Geometry: final body of the model. Coordinates: model frame, mm. A direction names the side the tool comes from. Give positions to 0.01 mm unless a question says otherwise; leave off trailing zeros. Order: outer loops, then holes, each group sorted by start corner. A loop starts at its lowest first (then second) coordinate and runs counter-clockwise, first axis right, second up. Notation, with made-up numbers: (34, -12) -> (48, -12) arc R9 cw to (48, 0) -> close; hole circle Ø11 at (-36, 50). An arc over 180 degrees is marked (long way). One line per question, with ' | ' between items.
Autodesk Inventor part; units mm, degrees
ref_plane "YZ Plane" through (0, 0, 0) normal (1, 0, 0) x (0, 1, 0)
ref_plane "XZ Plane" through (0, 0, 0) normal (0, 1, 0) x (-1, 0, 0)
ref_plane "XY Plane" through (0, 0, 0) normal (0, 0, 1) x (1, 0, 0)
sketch "Skizze1" plane through (0, 0, 0) normal (0, 0, 1) x (1, 0, 0)
  line L0 (0, 0) -> (0, 1.7)
  line L1 (0, 1.7) -> (-5, 1.7)
  line L2 (-5, 1.7) -> (-5, 0.2)
  line L3 (-5, 0.2) -> (-7.5, 0.2)
  line L4 (-7.5, 0.2) -> (-7.5, -1.3)
  line L5 (-7.5, -1.3) -> (-3.5, -1.3)
  line L6 (-3.5, -1.3) -> (-3.5, 0)
  line L7 (-3.5, 0) -> (0, 0)
  dimension "d0" = 4
  dimension "d1" = 1.5
  dimension "d2" = 2.5
  dimension "d3" = 3
  dimension "d4" = 5
  dimension "d5" = 1.7
extrude "Extrusion1" add sketch "Skizze1" along normal blind 30
mirror "Spiegeln1" about plane through (0, 0, 0) normal (1, 0, 0) of "Extrusion1"
sketch "Skizze2" plane through (-5, 1.7, 30) normal (0, 1, 0) x (1, 0, 0)
  circle A0 centre (5, 24) radius 2.25
  circle A1 centre (5, 6) radius 2.25
  line L0 (10, 30) -> (0, 30)
  line L1 (5, 30) -> (5, 24) construction
  line L2 (5, 6) -> (5, 0) construction
  line L3 (0, 0) -> (10, 0) construction
  dimension "d8" = 4.5
  dimension "d9" = 18
extrude "Extrusion2" add sketch "Skizze2" along normal blind 2.3
sketch "Skizze3" plane through (0, 4, 24) normal (0, 1, 0) x (1, 0, 0)
  circle A0 centre (0, 0) radius 2.25 construction
  circle A1 centre (0, 18) radius 2.25 construction
  point P0 (0, 24)
hole "Bohrung1" at (0, 4, 24) at (0, 4, 6) direction (0, -1, 0) diameter 2.459 end through all countersink diameter 3.5 countersink angle 90
properties part number "Igus Gleiter"
1) Section C-C on y = -0.55. Return loops of the section in (x, z).
Check result:
outline: (-7.5, 0) -> (-3.5, 0) -> (-3.5, 30) -> (-7.5, 30) -> close; (3.5, 0) -> (7.5, 0) -> (7.5, 30) -> (3.5, 30) -> close
2) Section D-D on z = 19.5. Return loops of the section in (x, y), plus the area to 3 significant figures.
Check result:
outline: (-7.5, -1.3) -> (-3.5, -1.3) -> (-3.5, 0) -> (3.5, 0) -> (3.5, -1.3) -> (7.5, -1.3) -> (7.5, 0.2) -> (5, 0.2) -> (5, 1.7) -> (-5, 1.7) -> (-5, 0.2) -> (-7.5, 0.2) -> close | area: 28.4 mm^2
3) Section B-B on z = 24. Return loops of the section in (x, y).
Check result:
outline: (-7.5, -1.3) -> (-3.5, -1.3) -> (-3.5, 0) -> (-1.23, 0) -> (-1.23, 3.48) -> (-1.75, 4) -> (-2.25, 4) -> (-2.25, 1.7) -> (-5, 1.7) -> (-5, 0.2) -> (-7.5, 0.2) -> close; (1.23, 0) -> (3.5, 0) -> (3.5, -1.3) -> (7.5, -1.3) -> (7.5, 0.2) -> (5, 0.2) -> (5, 1.7) -> (2.25, 1.7) -> (2.25, 4) -> (1.75, 4) -> (1.23, 3.48) -> close
4) Section A-A on x = 0. Return loops of the section in (y, z), plus the area to 3 significant figures.
Check result:
outline: (0, 0) -> (1.7, 0) -> (1.7, 3.75) -> (4, 3.75) -> (4, 4.25) -> (3.48, 4.77) -> (0, 4.77) -> close; (0, 7.23) -> (3.48, 7.23) -> (4, 7.75) -> (4, 8.25) -> (1.7, 8.25) -> (1.7, 21.75) -> (4, 21.75) -> (4, 22.25) -> (3.48, 22.77) -> (0, 22.77) -> close; (0, 25.23) -> (3.48, 25.23) -> (4, 25.75) -> (4, 26.25) -> (1.7, 26.25) -> (1.7, 30) -> (0, 30) -> close | area: 51.5 mm^2
5) Set-up query: faces 1 (the flat face through (5, 1, 15)), 2 (the flat face through (-3.5, -1, 15)), 3 (the cylindrical face through (1.21, 2.834, 7.897)), 4 (the flat face through (-6, 0.2, 15)). Return all of +Z, -Z, +X, -X, +Y, -Y with unobstructed straight access to the full face (end or side cutting, diameter ignored); none if empty.
Check result:
face 1: +Z, -Z, +X, +Y | face 2: +Z, -Z, -Y | face 3: +Y | face 4: +Z, -Z, -X, +Y
6) Pull-direction query (X, two-part tool) for faces 5 (the flat face through (-5, 1, 15)), 6 (the flat face through (6, 0.2, 15)), 7 (the cylindrical face through (-0.05, 1.72, 4.77)); classes: +X half, -X half, draft (parallel to the pull), parting line (faces both ways), or undercut.
Check result:
face 5: -X half | face 6: draft | face 7: undercut
7) Material intervals for probe 1 along Z at (x, y) = (0, 1.25); probe 2 along Z at (x, y) = (0, 2.5); probe 3 along X at (y, z) = (1.4, 6), sorted ascending. Write a range as from..to.
Check result:
probe 1: z = 0..4.77, 7.23..22.77, 25.23..30 | probe 2: z = 3.75..4.77, 7.23..8.25, 21.75..22.77, 25.23..26.25 | probe 3: x = -5..-1.23, 1.23..5
8) Contact query for flat-ended pins moving along their axis: pin 1 Ø1.2 at (x, z) = (-6, 18.5) entering from +Y; pin 2 Ø1.2 at (y, z) = (1.5, 18.5) entering from -X; pin 3 Ø1 at (x, z) = (1.5, 25.5) entering from -Y. Output: stop coordinate, or through.
Check result:
pin 1: stops at y = 0.2 | pin 2: stops at x = -5 | pin 3: stops at y = 0
